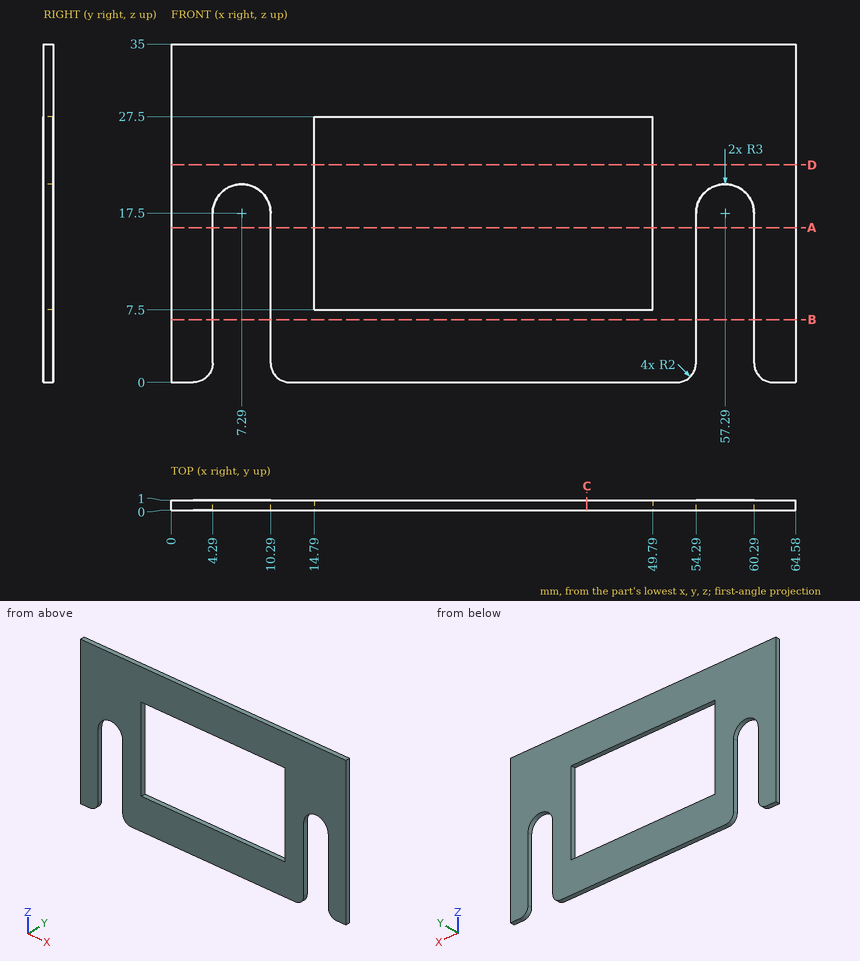
Geometry: see drawing. Coordinates: mm, zero at the bounding-box minimum. Give positions to 0.01 mm unless a question says otherwise; leave off trailing zeros. Write each loop counter-clockwise with the first axis right and the second up, starting at its lowest first coordinate (ties: lowest second). Pieces come first, ordered by that corner, then holes. Notation, with made-up numbers: (24, 67.25) -> (48, 67.25) arc R18 ccw to (48, 90.25) -> close; hole circle Ø5 at (30, 73.5). An arc over 180 degrees is marked (long way). Use one line per item in the form item = value. Start each with the question number.
1) Section query D-D on z = 22.5. Return the cut outline in (x, y).
2) Section query B-B on z = 6.5. Return the cut outline in (x, y), then the cut area to 3 significant figures.
3) Ray query, probe 1 along X at (y, z) = (0.3, 6.5); probe 2 along X at (y, z) = (0.8, 11); probe 3 along Z at (x, y) = (22, 0.15). Return the intervals inside material, ascending. Write a range as from..to.
4) Section query C-C on x = 43. Return the cut outline in (y, z), then the cut area to 3 significant figures.
5) Section query A-A on z = 16. Return the cut outline in (x, y), then the cut area to 3 significant figures.
Outcome:
q1.outline = (0, 0) -> (14.79, 0) -> (14.79, 1) -> (0, 1) -> close; (49.79, 0) -> (64.58, 0) -> (64.58, 1) -> (49.79, 1) -> close
q2.outline = (0, 0) -> (4.29, 0) -> (4.29, 1) -> (0, 1) -> close; (10.29, 0) -> (54.29, 0) -> (54.29, 1) -> (10.29, 1) -> close; (60.29, 0) -> (64.58, 0) -> (64.58, 1) -> (60.29, 1) -> close
q2.area = 52.6 mm^2
q3.probe_1 = 0..4.29, 10.29..54.29, 60.29..64.58
q3.probe_2 = 0..4.29, 10.29..14.79, 49.79..54.29, 60.29..64.58
q3.probe_3 = 0..7.5, 27.5..35
q4.outline = (0, 0) -> (1, 0) -> (1, 7.5) -> (0, 7.5) -> close; (0, 27.5) -> (1, 27.5) -> (1, 35) -> (0, 35) -> close
q4.area = 15.0 mm^2
q5.outline = (0, 0) -> (4.29, 0) -> (4.29, 1) -> (0, 1) -> close; (10.29, 0) -> (14.79, 0) -> (14.79, 1) -> (10.29, 1) -> close; (49.79, 0) -> (54.29, 0) -> (54.29, 1) -> (49.79, 1) -> close; (60.29, 0) -> (64.58, 0) -> (64.58, 1) -> (60.29, 1) -> close
q5.area = 17.6 mm^2
